Drawing for the job (mm, zero at the part's lowest x, y, z). Round coordinates to 2 decimals unless told otherwise and drop trailing zeros. Write each loop counter-clockwise with the first axis right and the second up, starting at its lowest first coordinate (ties: lowest second). Pieces come first, ordered by that corner, then holes. Notation, with made-up numbers: M 70,-27.5 L 115,-27.5 A31 cw 115,10.5 Z; hole C -37.5,-20.75 d1. An arc over 180 degrees is marked long. Use a Markdown table: item, result. Add a question column.
1) Wall check: probe 1 along X at (y, z) = (41.5, 0.15); probe 2 along Y at (x, z) = (5, 2.5); probe 3 along X at (y, z) = (28.5, 0.5). Give the ranges that are in metal, low to high.
2) Slice it at A-A on x = 5.5. Write the cut outline in (y, z), plus the area to 3 significant figures.
3) Drop flat-ended pins along their axis: P1, Ø1.5, axis at y = 13.5, z = 1, coming from the +X side; P2, Ø1.5, axis at x = 50, z = 1, coming from the -Y side; P3, Ø1, axis at x = 8.5, z = 0.5, coming from the +Y side. Give the stop position or say it passes through.
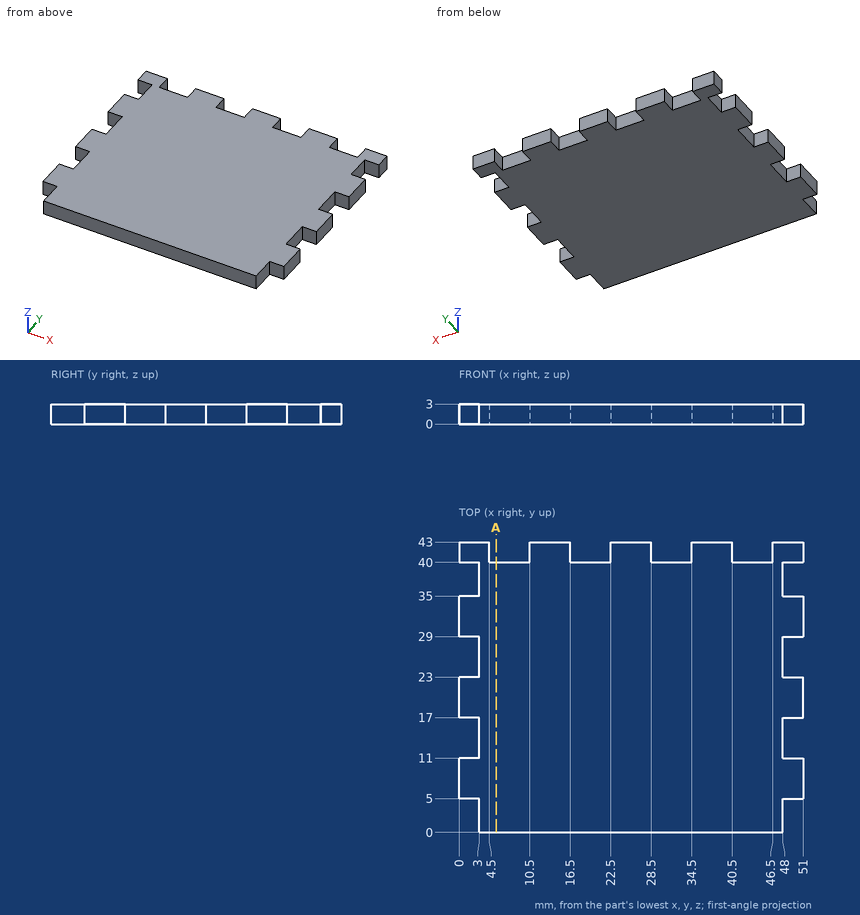
Entries:
| question | item | result |
|---|---|---|
| 1 | probe 1 | x = 0 to 4.5, 10.5 to 16.5, 22.5 to 28.5, 34.5 to 40.5, 46.5 to 51 |
| 1 | probe 2 | y = 0 to 40 |
| 1 | probe 3 | x = 3 to 48 |
| 2 | outline | M 0,0 L 40,0 L 40,3 L 0,3 Z |
| 2 | area | 120 mm^2 |
| 3 | P1 | stops at x = 48 |
| 3 | P2 | stops at y = 5 |
| 3 | P3 | stops at y = 40 |
